```python
from build123d import *

# Parameters (mm, degrees)
SCHIZZO1_R                   = 10.275
ESTRUSIONE_ESTRUSIONE1_DEPTH = 1.9
RACCORDO1_R                  = 0.5


with BuildPart() as part:
    # Schizzo1 → Estrusione-Estrusione1 (new, symmetric)
    with BuildSketch(Plane.XY):
        Polygon((-15.530722241, 0), (-7.765361121, -13.45), (7.765361121, -13.45), (15.530722241, 0), (7.765361121, 13.45), (-7.765361121, 13.45), align=None)
        with Locations(Location((0, 0, 0), (0, 0, 180))):
            Circle(SCHIZZO1_R, mode=Mode.SUBTRACT)
    extrude(amount=ESTRUSIONE_ESTRUSIONE1_DEPTH, both=True)

    # Raccordo1
    raccordo1_edges = [part.edges().sort_by_distance(p)[0] for p in [
        (0, -13.45, 1.9),
        (11.648041681, -6.725, 1.9),
        (11.648041681, 6.725, 1.9),
        (10.275, 0, -1.9),
        (10.275, 0, 1.9),
        (0, 13.45, 1.9),
        (-11.648041681, 6.725, 1.9),
        (0, 13.45, -1.9),
        (11.648041681, 6.725, -1.9),
        (11.648041681, -6.725, -1.9),
        (-11.648041681, -6.725, 1.9),
        (0, -13.45, -1.9),
        (-11.648041681, -6.725, -1.9),
        (-11.648041681, 6.725, -1.9),
    ]]
    fillet(raccordo1_edges, radius=RACCORDO1_R)


solid = part.part
```
CAD build for the part. Positions are in the model's coordinates, mm. Coordinates: 2 decimals unless noted, no trailing zeros. Loops run counter-clockwise (first coordinate to the right, second up) from the corner with the lowest first, then second, coordinate; pieces in that order, holes last. Notation, with made-up numbers: (73, -16.75) - (118, -16.75) arc R15 cw to (118, 12.25) - close; hole circle Ø10 at (63.5, 4.25). An arc over 180 degrees is marked (long way). Use CSV: the item, a comma, the result in double quotes. Start each with the question number.
Q1. Probe probe 1 along Y at (x, z) = (0, -0.7) (3 decimals); probe 2 along Y at (x, z) = (1.5, -0.5); probe 3 along X at (y, z) = (-9.25, 0.2). List the from-to ranges inside material, lowest first. Write a range as from..to.
Q2. Two-plate mould, pull along X, no slides. Class faces 1 (the flat face through (3, 11, 1.9)), 2 (the cylindrical face through (11.58, -6.56, -1.75)), 3 (the cylindrical face through (2.23, 10.03, -0.02)): +X half, -X half, draft (parallel to the pull), parting line (faces both ways), or undercut.
Q3. Cut at A-A, the plane x = 0. List the corners of the cut face in (y, z) (3 decimals), then the cut area to 3 significant figures.
Q4. Cut at B-B, the plane z = -0.7. List the corners of the cut face in (x, y) (3 decimals).
Q5. Drop a flat-ended pin along its axis: P1, Ø2, axis at y = -2, z = 0.5, coming from the -X side. Give the stop position or say it passes through.
Here are the results:
1,probe 1,"-13.45..-10.275, 10.275..13.45"
1,probe 2,"-13.45..-10.16, 10.16..13.45"
1,probe 3,"-10.19..-4.47, 4.47..10.19"
2,face 1,"draft"
2,face 2,"+X half"
2,face 3,"undercut"
3,outline,"(-13.45, -1.4) arc R0.5 ccw to (-12.95, -1.9) - (-10.775, -1.9) arc R0.5 ccw to (-10.275, -1.4) - (-10.275, 1.4) arc R0.5 ccw to (-10.775, 1.9) - (-12.95, 1.9) arc R0.5 ccw to (-13.45, 1.4) - close; (10.275, -1.4) arc R0.5 ccw to (10.775, -1.9) - (12.95, -1.9) arc R0.5 ccw to (13.45, -1.4) - (13.45, 1.4) arc R0.5 ccw to (12.95, 1.9) - (10.775, 1.9) arc R0.5 ccw to (10.275, 1.4) - close"
3,area,"23.7 mm2"
4,outline,"(-15.531, 0) - (-7.765, -13.45) - (7.765, -13.45) - (15.531, 0) - (7.765, 13.45) - (-7.765, 13.45) - close; hole circle Ø20.55 at (0, 0)"
5,P1,"x = -14.95"
